Could you check a few things on this drawing? It's one solid part, dimensions in mm from its lowest x, y, z. Coordinates: 2 decimals unless noted, no trailing zeros. Write each loop counter-clockwise with the first axis right and the second up, starting at its lowest first coordinate (ties: lowest second). Pieces come first, ordered by that corner, then holes. Notation, with made-up numbers: (75.25, 28.25) - (122.25, 28.25) arc R18 cw to (122.25, 36.25) - close; hole circle Ø3 at (24.25, -8). An arc over 180 degrees is marked (long way). Answer as a JSON object with one key per item and string values. Group by question number.
1) Please list where these lines run through material, in increasing order: line 1 along X through (y, z) = (14.25, 3.1); line 2 along Y through (x, z) = (34, 1.2).
2) If we section it at B-B (x = 43.5): Write out the boundary of the cut face in (y, z).
3) Will this pin go through, and if not, where does the flat tip stop? pin 1 Ø1.5 at (x, z) = (56, 1.5) entering from +Y.
4) If we section it at A-A (z = 1.2): Write out the boundary of the cut face in (x, y).
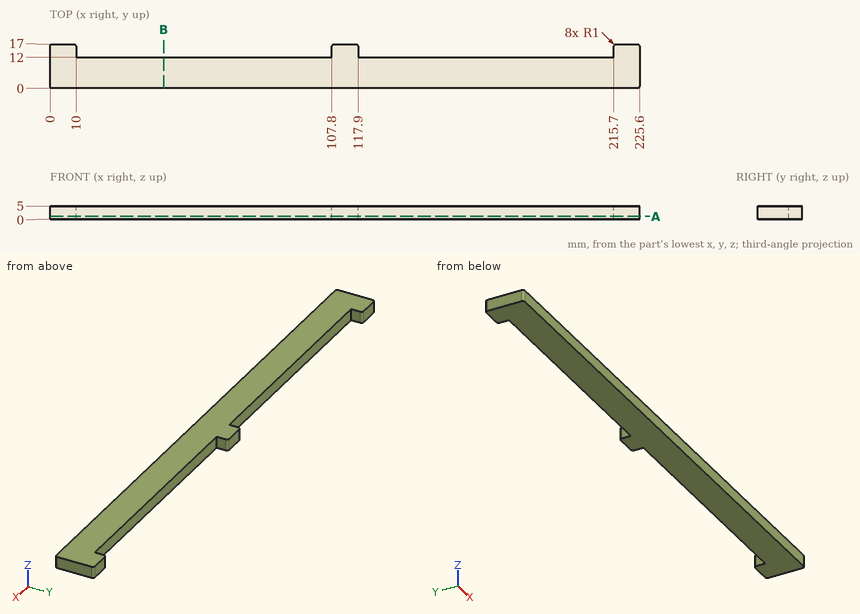
Here are the results:
{
 "1": {"line 1": "x = 0 to 10, 107.8 to 117.9, 215.7 to 225.6", "line 2": "y = 0 to 12"},
 "2": {"outline": "(0, 0) - (12, 0) - (12, 5) - (0, 5) - close"},
 "3": {"pin 1": "stops at y = 12"},
 "4": {"outline": "(0, 1) arc R1 ccw to (1, 0) - (224.6, 0) arc R1 ccw to (225.6, 1) - (225.6, 16) arc R1 ccw to (224.6, 17) - (216.7, 17) arc R1 ccw to (215.7, 16) - (215.7, 12) - (117.9, 12) - (117.9, 16) arc R1 ccw to (116.9, 17) - (108.8, 17) arc R1 ccw to (107.8, 16) - (107.8, 12) - (10, 12) - (10, 16) arc R1 ccw to (9, 17) - (1, 17) arc R1 ccw to (0, 16) - close"}
}
